Verification items for the finished model (mm, model axes). A direction names the side the tool comes from. Round coordinates to 2 decimals unless told otherwise and drop trailing zeros. Loops run counter-clockwise (first coordinate to the right, second up) from the corner with the lowest first, then second, coordinate; pieces in that order, holes last. Notation, with made-up numbers: (34, 60.25) -> (86, 60.25) arc R27 ccw to (86, 82.25) -> close; hole circle Ø8 at (81.25, 34.25). An arc over 180 degrees is marked (long way). Write item = value, one per line. Start each with the question number.
Autodesk Inventor part; units mm, degrees
ref_plane "YZ Plane" through (0, 0, 0) normal (1, 0, 0) x (0, 1, 0)
ref_plane "XZ Plane" through (0, 0, 0) normal (0, 1, 0) x (-1, 0, 0)
ref_plane "XY Plane" through (0, 0, 0) normal (0, 0, 1) x (1, 0, 0)
sketch "Sketch1" plane through (0, 0, 0) normal (0, 0, 1) x (1, 0, 0)
  line L0 (-12.7, 30.861) -> (12.7, 30.861)
  line L1 (12.7, 30.861) -> (12.7, -30.861)
  line L2 (12.7, -30.861) -> (-12.7, -30.861)
  line L3 (-12.7, -30.861) -> (-12.7, 30.861)
  line L4 (-12.7, 30.861) -> (12.7, -30.861) construction
  line L5 (12.7, 30.861) -> (-12.7, -30.861) construction
  point P0 (0, 0)
  dimension "d0" = 25.4
  dimension "d1" = 61.722
extrude "Extrusion1" add sketch "Sketch1" along normal blind 1.397
sketch "Sketch2" plane through (0, 0, 1.397) normal (0, 0, 1) x (1, 0, 0)
  line L0 (-10.16, -30.861) -> (10.16, -30.861)
  line L1 (10.16, -30.861) -> (10.16, 22.479)
  line L2 (10.16, 22.479) -> (-10.16, 22.479)
  line L3 (-10.16, 22.479) -> (-10.16, -30.861)
  line L4 (-12.7, -30.861) -> (12.7, -30.861)
  point P0 (0, 0)
  point P1 (0, -30.861)
  dimension "d4" = 20.32
  dimension "d5" = 53.34
extrude "Extrusion2" cut sketch "Sketch2" against normal through all
sketch "Sketch3" plane through (12.7, -30.861, 0) normal (1, 0, 0) x (0, 0, -1)
  line L0 (0, 61.722) -> (0, 0)
  line L1 (0, 61.722) -> (-1.397, 61.722)
  line L2 (-1.397, 0) -> (-1.397, 61.722)
  line L3 (0, 0) -> (-1.397, 0)
  line L4 (-1.397, 0) -> (-1.905, 0)
  line L5 (-1.397, 0) -> (-1.397, 1.27)
  line L6 (-1.397, 53.34) -> (-1.397, 0)
  line L7 (-1.651, 1.27) -> (-1.397, 1.27)
  line L8 (-1.651, 1.27) -> (-1.905, 0)
  point P0 (0, 30.861)
  dimension "d8" = 0.508
  dimension "d9" = 1.27
  dimension "d10" = 0.254
ref_plane "Work Plane1" through (0, 0, 1.651) normal (0, 0, 1) x (1, 0, 0)
sketch "Sketch6" plane through (0, 0, 1.651) normal (0, 0, 1) x (1, 0, 0)
  line L0 (12.7, -29.591) -> (12.7, -30.861)
  line L1 (12.7, -30.861) -> (12.7, 30.861)
  line L2 (12.7, -30.226) -> (10.795, -30.226)
  line L3 (10.16, -30.861) -> (12.7, -30.861)
  line L4 (10.16, 22.479) -> (10.16, -30.861)
  line L5 (10.795, -30.226) -> (10.795, 23.114)
  line L6 (10.795, 23.114) -> (-10.795, 23.114)
  line L7 (-10.795, 23.114) -> (-10.795, -30.226)
  line L8 (-10.795, -30.226) -> (-12.7255, -30.226)
  line L9 (-12.7, -30.861) -> (-10.16, -30.861)
  line L10 (-10.16, -30.861) -> (-10.16, 22.479)
  line L11 (-10.16, 22.479) -> (10.16, 22.479)
  point P0 (0, 0)
  dimension "d12" = 0.635
  dimension "d13" = 0.635
  dimension "d14" = 0.635
  dimension "d15" = 0.635
  dimension "d16" = 0.635
sweep "Sweep1" add profiles "Sketch3" path "Sketch6" path curves L2 L5 L6 L7 L8 contours L4 L8 L7 L2
properties part number "door"
(1) Access from +Z, -Z, +X, -X, +Y, -Y to the whole of each face (thin tool, end or side, straight path). Record for faces 4 (the flat face through (0, 22.479, 1)), 5 (the flat face through (11.694, -30.217, 1.776)), 6 (the flat face through (-11.746, -30.217, 1.776)), 7 (the flat face through (12.7, 0, 1)).
(2) Draft check along X on faces 1 (the flat face through (-11, -30.861, 1)), 2 (the flat face through (10.804, -3.174, 1.776)), 3 (the flat face through (-10.16, -4, 1)). Enter one of: +X half, -X half, draft (parallel to the pull), parting line (faces both ways), or undercut.
(3) Section check D-D on y = 27.5. Enter the section's corners in (x, z), then the cut area to 3 significant figures.
(4) Depth check by flat-ended pin: pin 1 Ø1.1 at (y, z) = (13.5, 0.5) entering from -X; pin 2 Ø4 at (x, y) = (-9, -10) entering from -Z. Enter the tip coordinate at first touch or a pass-through.
(5) Section check C-C on x = 2.75. Enter the section's corners in (y, z) (3 decimals), then the cut area to 3 significant figures.
(6) Scan lines: line 1 (X direction, y = -5, z = 1.6); line 2 (X direction, y = -1, z = 0.25); line 3 (Y direction, x = 5, z = 0.85). Record each from-to range of solid material in increasing order. Write a range as [from, to].
(7) Section check B-B on z = 0.45. Enter the section's corners in (x, y).
(8) Section check A-A on y = -16.5. Enter the section's corners in (x, z) (3 decimals).
Computed values:
q1.face_4 = +Z, -Z, -Y
q1.face_5 = +Z, +X, +Y
q1.face_6 = +Z, -X, +Y
q1.face_7 = +Z, -Z, +X, +Y, -Y
q2.face_1 = draft
q2.face_2 = +X half
q2.face_3 = undercut
q3.outline = (-12.7, 0) -> (12.7, 0) -> (12.7, 1.4) -> (-12.7, 1.4) -> close
q3.area = 35.5 mm²
q4.pin_1 = -12.7
q4.pin_2 = 0
q5.outline = (22.479, 0) -> (30.861, 0) -> (30.861, 1.397) -> (23.749, 1.397) -> (23.749, 1.651) -> (22.479, 1.905) -> close
q5.area = 12.2 mm²
q6.line_1 = [-11.43, -10.16], [10.16, 11.43]
q6.line_2 = [-12.7, -10.16], [10.16, 12.7]
q6.line_3 = [22.48, 30.86]
q7.outline = (-12.7, -30.86) -> (-10.16, -30.86) -> (-10.16, 22.48) -> (10.16, 22.48) -> (10.16, -30.86) -> (12.7, -30.86) -> (12.7, 30.86) -> (-12.7, 30.86) -> close
q8.outline = (-12.7, 0) -> (-10.16, 0) -> (-10.16, 1.905) -> (-11.43, 1.651) -> (-11.43, 1.397) -> (-12.7, 1.397) -> close; (10.16, 0) -> (12.7, 0) -> (12.7, 1.397) -> (11.43, 1.397) -> (11.43, 1.651) -> (10.16, 1.905) -> close
